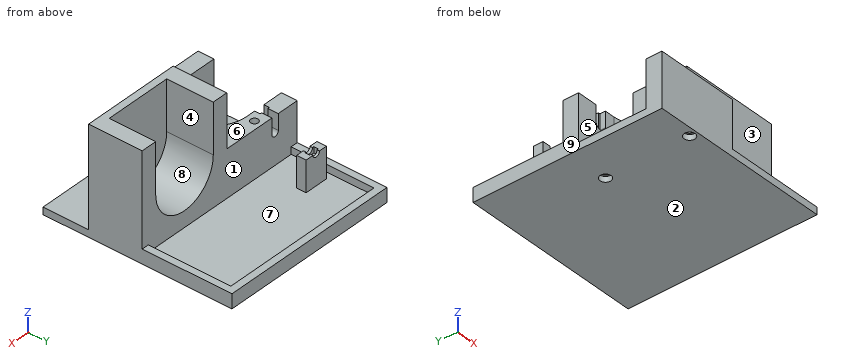
from build123d import *

# Parameters (mm, degrees)
SKETCH_W        = 77
SKETCH_H        = 80
PAD_DEPTH       = 3
SKETCH001_W     = 35
SKETCH001_H     = 42
PAD001_DEPTH    = 19.7
POCKET_DEPTH    = 19.7
SKETCH003_W     = 42
SKETCH003_H     = 22.7
PAD002_DEPTH    = 42
POCKET001_DEPTH = 19.7
SKETCH006_R     = 1.6
POCKET002_DEPTH = 8
SKETCH007_R     = 2.3
POCKET003_DEPTH = 2.3
SKETCH008_W     = 10
SKETCH008_H     = 4
PAD003_DEPTH    = 13
POCKET004_DEPTH = 4
POCKET005_DEPTH = 6.7
SKETCH011_W     = 4.4
SKETCH011_H     = 1.9
POCKET006_DEPTH = 2.5
SKETCH012_R     = 1.6
POCKET007_DEPTH = 22.701
PAD004_DEPTH    = 3
SKETCH014_R     = 2.3
POCKET008_DEPTH = 2.3


with BuildPart() as part:
    # Sketch → Pad (new body)
    with BuildSketch(Plane.XY):
        with Locations((4.24216, 5.423944)):
            Rectangle(SKETCH_W, SKETCH_H)
    extrude(amount=PAD_DEPTH)

    # Sketch001 → Pad001 (new body)
    with BuildSketch(Plane.XY.offset(3)):
        with Locations((-16.75784, -13.576056)):
            Rectangle(SKETCH001_W, SKETCH001_H)
    extrude(amount=PAD001_DEPTH)

    # Sketch002 → Pocket (cut)
    with BuildSketch(Plane.XY.offset(22.7)):
        with BuildLine():
            ThreePointArc((-16.75784, -27.876056), (-2.45784, -13.576056), (-16.75784, 0.723944))
            Line((-16.75784, 0.723944), (-34.25784, 0.723944))
            Line((-34.25784, -27.876057), (-34.25784, 0.723944))
            Line((-16.75784, -27.876056), (-34.25784, -27.876057))
        make_face()
    extrude(amount=-POCKET_DEPTH, mode=Mode.SUBTRACT)

    # Sketch003 → Pad002 (new body)
    with BuildSketch(Plane.XY.offset(3)):
        with Locations((21.74216, -3.926056)):
            Rectangle(SKETCH003_W, SKETCH003_H)
    extrude(amount=PAD002_DEPTH)

    # Sketch004 → Pocket001 (cut)
    with BuildSketch(Plane(origin=(0, 7.423944, 0), x_dir=(-1, 0, 0), z_dir=(0, 1, 0))):
        with BuildLine():
            ThreePointArc((-36.04216, 24), (-21.74216, 9.7), (-7.44216, 24))
            Line((-7.44216, 24), (-7.44216, 45))
            Line((-36.04216, 45), (-7.44216, 45))
            Line((-36.04216, 24), (-36.04216, 45))
        make_face()
    extrude(amount=-POCKET001_DEPTH, mode=Mode.SUBTRACT)

    # Sketch006 → Pocket002 (cut)
    with BuildSketch(Plane(origin=(0, 7.423944, 0), x_dir=(-1, 0, 0), z_dir=(0, 1, 0))):
        with Locations((23.25784, 16)):
            Circle(SKETCH006_R)
    extrude(amount=-POCKET002_DEPTH, mode=Mode.SUBTRACT)

    # Sketch007 → Pocket003 (cut)
    with BuildSketch(Plane.XZ.offset(-0.723944)):
        with Locations((-23.25784, 16)):
            Circle(SKETCH007_R)
    extrude(amount=-POCKET003_DEPTH, mode=Mode.SUBTRACT)

    # Sketch008 → Pad003 (new body)
    with BuildSketch(Plane.XY.offset(3)):
        with Locations((-23.25784, 22.823944)):
            Rectangle(SKETCH008_W, SKETCH008_H)
    extrude(amount=PAD003_DEPTH)

    # Sketch009 → Pocket004 (cut)
    with BuildSketch(Plane(origin=(0, 24.823944, 0), x_dir=(-1, 0, 0), z_dir=(0, 1, 0))):
        with BuildLine():
            ThreePointArc((21.65784, 16), (23.25784, 14.4), (24.85784, 16))
            Line((21.65784, 16), (24.85784, 16))
        make_face()
    extrude(amount=-POCKET004_DEPTH, mode=Mode.SUBTRACT)

    # Sketch010 → Pocket005 (cut)
    with BuildSketch(Plane.XY.offset(22.7)):
        Polygon((-24.85784, 7.423944), (-21.65784, 7.423944), (-21.65784, 3.023944), (-20.95784, 3.023944), (-20.95784, 0.723944), (-25.55784, 0.723944), (-25.55784, 3.023944), (-24.85784, 3.023944), align=None)
    extrude(amount=-POCKET005_DEPTH, mode=Mode.SUBTRACT)

    # Sketch011 → Pocket006 (cut)
    with BuildSketch(Plane.XY.offset(16)):
        with Locations((-23.25784, 22.873944)):
            Rectangle(SKETCH011_W, SKETCH011_H)
    extrude(amount=-POCKET006_DEPTH, mode=Mode.SUBTRACT)

    # Sketch012 → Pocket007 (cut, through all)
    with BuildSketch(Plane.XY.offset(22.7)):
        with Locations((-16.75784, -31.376056)):
            Circle(SKETCH012_R)
        with Locations((-16.75784, 4.223944)):
            Circle(SKETCH012_R)
    extrude(amount=-POCKET007_DEPTH, mode=Mode.SUBTRACT)

    # Sketch013 → Pad004 (new body)
    with BuildSketch(Plane.XY.offset(3)):
        Polygon((-34.25784, 7.423944), (-34.25784, 45.423944), (42.74216, 45.423944), (42.74216, 7.423944), (39.74216, 7.423944), (39.74216, 42.423944), (-31.25784, 42.423944), (-31.25784, 7.423944), align=None)
    extrude(amount=PAD004_DEPTH)

    # Sketch014 → Pocket008 (cut)
    with BuildSketch(Plane(origin=(0, 0, 0), x_dir=(1, 0, 0), z_dir=(0, 0, -1))):
        with Locations((-16.75784, 31.376056)):
            Circle(SKETCH014_R)
        with Locations((-16.75784, -4.223944)):
            Circle(SKETCH014_R)
    extrude(amount=-POCKET008_DEPTH, mode=Mode.SUBTRACT)


solid = part.part
Verification items for the finished model (mm, model axes). Face numbers are marked on the shaded views. A direction names the side the tool comes from. Round coordinates to 2 decimals unless told otherwise and drop trailing zeros. Loops run counter-clockwise (first coordinate to the right, second up) from the corner with the lowest first, then second, coordinate; pieces in that order, holes last. Notation, with made-up numbers: (5, 79) - (51, 79) arc R18 ccw to (51, 88) - close; hole circle Ø3 at (66.5, 55.5). An arc over 180 degrees is marked (long way). Use a Markdown table: item, result. Add a question column.
1. Thickness scan on probe 1 along X at (y, z) = (2.5, 30.5); probe 2 along X at (y, z) = (24.5, 3.5); probe 3 along X at (y, z) = (4, 17). Record the ranges inside material, lowest first. Write a range as [from, to].
2. Section check D-D, the plane y = 34. Record the boundary of the cut face in (x, z).
3. Section check C-C, the plane x = 11. Record the boundary of the cut face in (y, z), plus the area to 3 significant figures.
4. Section check A-A, the plane z = 19. Record the boundary of the cut face in (x, y).
5. Release check for a two-part mould opening along X. For the marked faces 6, 7, 8 and 9 record: released by +X, released by -X, zero draft, split by the parting line, or undercut.
6. Gauge pin test, flat ends, axial feed: pin 1 (19 mm diameter, centred on x = -23, z = 14, fed in from +Y); pin 2 (10 mm diameter, centred on x = -17, z = 23, fed in from +Y); pin 3 (4 mm diameter, centred on x = -17, z = 12, fed in from +Y); pin 4 (2 mm diameter, centred on y = 23, z = 10, fed in from -X). Record the tip position at first contact, or that the pin passes through.
7. Access from +Z, -Z, +X, -X, +Y, -Y to the whole of each face (thin tool, end or side, straight path). Record for the marked faces 1, 2, 3, 4 and 5.
8. Section check B-B, the plane z = 28. Record the boundary of the cut face in (x, y), plus the area to 3 significant figures.
Checks:
| question | item | result |
|---|---|---|
| 1 | probe 1 | x = [0.74, 7.44], [36.04, 42.74] |
| 1 | probe 2 | x = [-34.26, -31.26], [-28.26, -18.26], [39.74, 42.74] |
| 1 | probe 3 | x = [-34.26, -24.86], [-21.66, -18.34], [-15.17, 9.27], [34.21, 42.74] |
| 2 | outline | (-34.26, 0) - (42.74, 0) - (42.74, 6) - (39.74, 6) - (39.74, 3) - (-31.26, 3) - (-31.26, 6) - (-34.26, 6) - close |
| 3 | outline | (-34.58, 0) - (45.42, 0) - (45.42, 6) - (42.42, 6) - (42.42, 3) - (7.42, 3) - (7.42, 14.56) - (-12.28, 14.56) - (-12.28, 45) - (-15.28, 45) - (-15.28, 3) - (-34.58, 3) - close |
| 3 | area | 603 mm^2 |
| 4 | outline | (-34.26, -34.58) - (0.74, -34.58) - (0.74, -15.28) - (42.74, -15.28) - (42.74, 7.42) - (35.14, 7.42) - (35.14, -12.28) - (8.34, -12.28) - (8.34, 7.42) - (-21.66, 7.42) - (-21.66, 3.02) - (-20.96, 3.02) - (-20.96, 0.72) - (-16.76, 0.72) arc R14.3 cw to (-16.76, -27.88) - (-34.26, -27.88) - close; (-34.26, 0.72) - (-25.56, 0.72) - (-25.56, 3.02) - (-24.86, 3.02) - (-24.86, 7.42) - (-34.26, 7.42) - close; hole circle Ø3.2 at (-16.76, -31.38); hole circle Ø3.2 at (-16.76, 4.22) |
| 5 | face 6 | zero draft |
| 5 | face 7 | undercut |
| 5 | face 8 | undercut |
| 5 | face 9 | released by -X |
| 6 | pin 1 | stops at y = 45.42 |
| 6 | pin 2 | stops at y = 7.42 |
| 6 | pin 3 | stops at y = 24.82 |
| 6 | pin 4 | stops at x = -28.26 |
| 7 | face 1 | +Z |
| 7 | face 2 | -Z, +X, -X, +Y, -Y |
| 7 | face 3 | +Z, +X, -Y |
| 7 | face 4 | +Z, +Y |
| 7 | face 5 | +Z, -X |
| 8 | outline | (0.74, -15.28) - (42.74, -15.28) - (42.74, 7.42) - (36.04, 7.42) - (36.04, -12.28) - (7.44, -12.28) - (7.44, 7.42) - (0.74, 7.42) - close |
| 8 | area | 390 mm^2 |
